Geometry: final body of the model. Coordinates: model frame, mm. A direction names the side the tool comes from. Coordinates: 2 decimals unless noted, no trailing zeros. Write each loop counter-clockwise with the first axis right and the second up, starting at its lowest first coordinate (ties: lowest second). Pieces come first, ordered by that corner, then holes. Notation, with made-up numbers: M 60,59.25 L 80,59.25 A28 cw 80,84.25 Z; hole C 6,-40 d7. An arc over 180 degrees is marked long. Write item = value, one per line. Start each with the question number.
Item 1: Reachability of faces 1 (the flat face through (29, 88, 5)), 2 (the flat face through (59, 44, 5)), 3 (the flat face through (-13, 46, -13)), 4 (the flat face through (29, 47, -2)) from +Z, -Z, +X, -X, +Y, -Y: full face, straight path, thin tool, end or side. Return the list, or none.
Item 2: Pull-direction query (X, two-part tool) for faces 5 (the cylindrical face through (-9, 47, -24)), 6 (the flat face through (29, 0, 5)), 7 (the flat face through (29, 46, 2)), 8 (the flat face through (0, 44, 5)); classes: +X half, -X half, draft (parallel to the pull), parting line (faces both ways), or undercut.
Item 3: Section C-C on x = 32. Output: boundary loops of the cut face in (y, z), plus the area to 3 significant figures.
Item 4: Section B-B on z = -14.5. Output: boundary loops of the cut face in (x, y), plus the area to 3 significant figures.
Item 5: First-contact query: pin 1 Ø5 at (x, z) = (16.5, 5.5) entering from +Y; pin 2 Ø10 at (x, z) = (-1, -16) entering from +Y; pin 3 Ø1.6 at (x, y) = (25, 1) entering from +Z. Flat tips, straight axial feed; report the tip coordinate or a pass-through.
Item 6: Section A-A on y = 54. Output: boundary loops of the cut face in (x, z).
Item 7: Ray query, L1, parallel to X at y = 36.5, z = -8; L2, parallel to Z at x = 11, y = 87; L3, parallel to Z at x = -6.5, y = 60. Return the intervals inside material, ascending. Write a range as [from, to].
from build123d import *

# Parameters (mm, degrees)
BOX_W           = 59
BOX_H           = 90
BOX_DEPTH       = 8
SKETCH_W        = 55
SKETCH_H        = 86
POCKET_DEPTH    = 6
POCKET001_DEPTH = 2
SKETCH006_W     = 85
SKETCH006_H     = 100
PAD002_DEPTH    = 27
POCKET004_DEPTH = 98
FILLET_R        = 1.5
FILLET002_R     = 1.5


with BuildPart() as part:
    # Box → Box (join)
    with BuildSketch(Plane.XY):
        with Locations((29.5, 45)):
            Rectangle(BOX_W, BOX_H)
    extrude(amount=BOX_DEPTH)

    # Sketch (on Face6 of Box) → Pocket (cut)
    with BuildSketch(Plane.XY.offset(8)):
        with Locations((29.5, 45)):
            Rectangle(SKETCH_W, SKETCH_H)
    extrude(amount=-POCKET_DEPTH, mode=Mode.SUBTRACT)

    # Sketch001 (on Face2 of Pocket) → Pocket001 (cut)
    with BuildSketch(Plane.XZ):
        with BuildLine():
            Line((28.5, 8), (28.5, 7))
            ThreePointArc((26.5, 5), (27.914214, 5.585786), (28.5, 7))
            Line((26.5, 5), (21.5, 5))
            ThreePointArc((19.5, 7), (20.085786, 5.585786), (21.5, 5))
            Line((19.5, 7), (19.5, 8))
            Line((19.5, 8), (28.5, 8))
        make_face()
    extrude(amount=-POCKET001_DEPTH, mode=Mode.SUBTRACT)

    # Sketch006 (on Face5 of Pocket001) → Pad002 (join)
    with BuildSketch(Plane(origin=(0, 0, 0), x_dir=(1, 0, 0), z_dir=(0, 0, -1))):
        with Locations((29.5, -45)):
            Rectangle(SKETCH006_W, SKETCH006_H)
    extrude(amount=PAD002_DEPTH)

    # Sketch007 (on Face18 of Pad002) → Pocket004 (cut)
    with BuildSketch(Plane(origin=(0, 95, 0), x_dir=(-1, 0, 0), z_dir=(0, 1, 0))):
        with BuildLine():
            Line((-70, -7), (-70, -20))
            ThreePointArc((-70, -20), (-68.535534, -23.535534), (-65, -25))
            Line((-65, -25), (6, -25))
            ThreePointArc((6, -25), (9.535534, -23.535534), (11, -20))
            Line((11, -20), (11, -7))
            ThreePointArc((11, -7), (9.535534, -3.464466), (6, -2))
            Line((6, -2), (-65, -2))
            ThreePointArc((-65, -2), (-68.535534, -3.464466), (-70, -7))
        make_face()
    extrude(amount=-POCKET004_DEPTH, mode=Mode.SUBTRACT)

    # Fillet
    fillet_edges = [part.edges().sort_by_distance(p)[0] for p in [
        (0, 0, 4),
        (-13, -5, -13.5),
        (72, -5, -13.5),
        (59, 0, 4),
        (0, 90, 4),
        (-13, 95, -13.5),
        (59, 90, 4),
        (72, 95, -13.5),
    ]]
    fillet(fillet_edges, radius=FILLET_R)

    # Fillet002
    fillet002_edges = [part.edges().sort_by_distance(p)[0] for p in [
        (59, 45, 0),
        (72, 45, 0),
        (72, 45, -27),
    ]]
    fillet(fillet002_edges, radius=FILLET002_R)


solid = part.part
Responses:
q1.face_1 = +Z
q1.face_2 = +Z, +X, +Y, -Y
q1.face_3 = +Z, -Z, -X, +Y, -Y
q1.face_4 = +Y
q2.face_5 = undercut
q2.face_6 = draft
q2.face_7 = undercut
q2.face_8 = -X half
q3.outline = M -5,-25.5 A1.5 ccw -3.5,-27 L 93.5,-27 A1.5 ccw 95,-25.5 L 95,-25 L -3,-25 L -3,-2 L 95,-2 L 95,-1.5 A1.5 ccw 93.5,0 L 91.5,0 A1.5 cw 90,1.5 L 90,8 L 88,8 L 88,2 L 2,2 L 2,8 L 0,8 L 0,1.5 A1.5 cw -1.5,0 L -3.5,0 A1.5 ccw -5,-1.5 Z
q3.area = 649 mm²
q4.outline = M -13,-3.5 A1.5 ccw -11.5,-5 L 70.5,-5 A1.5 ccw 72,-3.5 L 72,93.5 A1.5 ccw 70.5,95 L 70,95 L 70,-3 L -11,-3 L -11,95 L -11.5,95 A1.5 ccw -13,93.5 Z
q4.area = 560 mm²
q5.pin_1 = 90
q5.pin_2 = -3
q5.pin_3 = 5
q6.outline = M -13,-25.5 A1.5 ccw -11.5,-27 L 70.5,-27 A1.5 ccw 72,-25.5 L 72,-1.5 A1.5 ccw 70.5,0 L 60.5,0 A1.5 cw 59,1.5 L 59,8 L 57,8 L 57,2 L 2,2 L 2,8 L 0,8 L 0,1.5 A1.5 cw -1.5,0 L -11.5,0 A1.5 ccw -13,-1.5 Z; hole M -11,-20 A5 ccw -6,-25 L 65,-25 A5 ccw 70,-20 L 70,-7 A5 ccw 65,-2 L -6,-2 A5 ccw -11,-7 Z
q7.L1 = [-13, -11], [70, 72]
q7.L2 = [-27, -25], [-2, 2]
q7.L3 = [-27, -24.97], [-2.03, 0]
